from build123d import *

# Parameters (mm, degrees)
F1_DEPTH = 90
F2_T     = -1.5
F4_DEPTH = 90.001
F6_DEPTH = 90


with BuildPart() as f1:
    # F0 (on Front) → F1 (new body)
    with BuildSketch(Plane.XZ):
        with BuildLine():
            ThreePointArc((40, -7.5), (47.5, 0), (40, 7.5))
            Line((40, 7.5), (-40, 7.5))
            ThreePointArc((-40, 7.5), (-47.5, 0), (-40, -7.5))
            Line((-40, -7.5), (40, -7.5))
        make_face()
    extrude(amount=F1_DEPTH)

    # F2
    f2_openings = [f1.faces().sort_by_distance(p)[0] for p in [
        (0, -90, 0),
        (0, 0, 0),
    ]]
    offset(amount=F2_T, openings=f2_openings)

    # F3 (on Front) → F4 (cut, through all)
    with BuildSketch(Plane.XZ):
        with BuildLine():
            ThreePointArc((40, 6), (46, 0), (40, -6))
            Line((40, -6), (-40, -6))
            Line((-40, -6), (-40, -7.5))
            Line((-40, -7.5), (40, -7.5))
            ThreePointArc((40, -7.5), (47.5, 0), (40, 7.5))
            Line((40, 7.5), (40, 6))
        make_face()
    extrude(amount=F4_DEPTH, mode=Mode.SUBTRACT)

    # F5 (on Front) → F6 (join, through all)
    with BuildSketch(Plane.XZ):
        with BuildLine():
            Line((34.257359, -6), (40, -6))
            ThreePointArc((40, -6), (46, 0), (40, 6))
            Line((40, 6), (34.257359, 6))
            Line((34.257359, 6), (34.257359, 1.5))
            Line((34.257359, 1.5), (35.757359, 1.5))
            ThreePointArc((35.757359, 1.5), (44.5, 0), (35.757359, -1.5))
            Line((35.757359, -1.5), (34.257359, -1.5))
            Line((34.257359, -1.5), (34.257359, -6))
        make_face()
    extrude(amount=F6_DEPTH)


solid = f1.part
Geometry check sheet. Reference: the model listing, model coordinates, mm. A direction names the side the tool comes from. Round coordinates to 2 decimals unless told otherwise and drop trailing zeros. Loops run counter-clockwise (first coordinate to the right, second up) from the corner with the lowest first, then second, coordinate; pieces in that order, holes last. Notation, with made-up numbers: (45.25, 75) -> (101.25, 75) arc R22 cw to (101.25, 86) -> close; hole circle Ø4 at (67, -26). An arc over 180 degrees is marked (long way). Answer as a JSON object with one key per item and string values. Group by question number.
Item 1: Release check for a two-part mould opening along X. For faces 1 (the face through (46, -44, 0)), 2 (the face through (-47.5, -44.37, 0.16)), 3 (the face through (44.497, -44.37, 0.176)), 4 (the face through (-0.97, 0, 6.15)) record: pulls with the +X half, pulls with the -X half, needs draft (parallel to the pull), parting line crosses it, or undercut.
Item 2: Cross-section at B-B, the plane y = -28. Record the cut outline in (x, z), plus the area to 3 significant figures.
Item 3: Depth check by flat-ended pin: pin 1 Ø7 at (x, z) = (40, 0) entering from +Y; pin 2 Ø1.2 at (y, z) = (-44, 7) entering from +X; pin 3 Ø8 at (x, y) = (-25, -21.5) entering from -Z; pin 4 Ø1.3 at (y, z) = (-67, -4) entering from -X. Enter the tip coordinate at first touch or a pass-through.
Item 4: Thickness scan on line 1 along X through (y, z) = (-12, -4); line 2 along X through (y, z) = (-62.5, 0); line 3 along X through (y, z) = (-28, -3). Record the ranges inside material, lowest first.
Item 5: Cross-section at A-A, the plane z = 0. Record the cut outline in (x, y), plus the area to 3 significant figures.
Item 6: Cross-section at C-C, the plane x = -25. Record the cut outline in (y, z).
Item 7: Set-up check for faces 5 (the face through (-46, -44, 0)), 6 (the face through (37, -44, -6)), 7 (the face through (34.257, -44, -4)), 8 (the face through (-0.97, -90, 6.15)): record each of +Z, -Z, +X, -X, +Y, -Y from which the full face is reachable in a straight line by a thin tool's end or side.
Determined:
{
 "1": {"face 1": "pulls with the +X half", "face 2": "pulls with the -X half", "face 3": "undercut", "face 4": "needs draft"},
 "2": {"outline": "(-40, -7.5) -> (-40, -6) arc R6 cw to (-40, 6) -> (34.26, 6) -> (34.26, 1.5) -> (35.76, 1.5) arc R4.5 cw (long way) to (35.76, -1.5) -> (34.26, -1.5) -> (34.26, -6) -> (40, -6) arc R6 ccw to (40, 6) -> (40, 7.5) -> (-40, 7.5) arc R7.5 ccw to start", "area": "210 mm²"},
 "3": {"pin 1": "passes through", "pin 2": "stops at x = 40", "pin 3": "stops at z = 6", "pin 4": "stops at x = -46.71"},
 "4": {"line 1": "x = -46.34 to -44.47, 34.26 to 37.94, 42.06 to 44.47", "line 2": "x = -47.5 to -46, 44.5 to 46", "line 3": "x = -46.87 to -45.2, 34.26 to 36.65, 43.35 to 45.2"},
 "5": {"outline": "(-47.5, -90) -> (-46, -90) -> (-46, 0) -> (-47.5, 0) -> close; (44.5, -90) -> (46, -90) -> (46, 0) -> (44.5, 0) -> close", "area": "270 mm²"},
 "6": {"outline": "(-90, 6) -> (0, 6) -> (0, 7.5) -> (-90, 7.5) -> close"},
 "7": {"face 5": "+Y, -Y", "face 6": "-Z, +X, +Y, -Y", "face 7": "-Z, +Y, -Y", "face 8": "+Z, -Z, +X, -X, -Y"}
}
